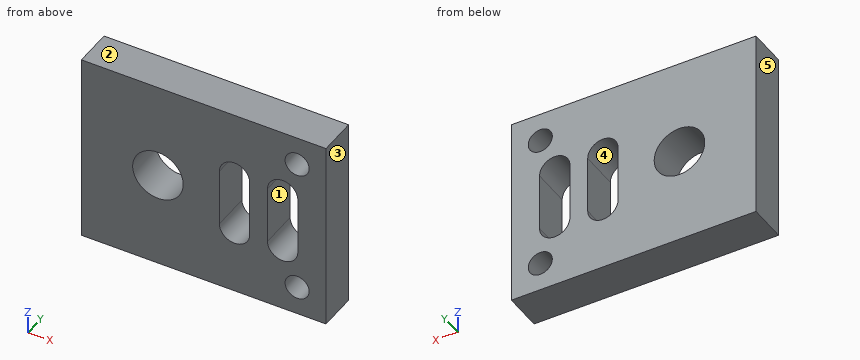
```python
from build123d import *

# Parameters (mm, degrees)
SKETCH1_W           = 25.4
SKETCH1_H           = 20
SKETCH1_R           = 1.25
SKETCH1_R_2         = 2.625
BOSS_EXTRUDE1_DEPTH = 4


with BuildPart() as part:
    # Sketch1 → Boss-Extrude1 (new body)
    with BuildSketch(Plane(origin=(0, 0, 0), x_dir=(1, 0, 0), z_dir=(0, 1, 0))):
        with Locations((12.7, 10)):
            Rectangle(SKETCH1_W, SKETCH1_H)
        with Locations((22.4, 17)):
            Circle(SKETCH1_R, mode=Mode.SUBTRACT)
        with Locations((7.95, 10)):
            Circle(SKETCH1_R_2, mode=Mode.SUBTRACT)
        with Locations((22.4, 3)):
            Circle(SKETCH1_R, mode=Mode.SUBTRACT)
        with BuildLine():
            Line((19.325, 7), (19.325, 13))
            ThreePointArc((19.325, 13), (20.9, 14.575), (22.475, 13))
            Line((22.475, 13), (22.475, 7))
            ThreePointArc((22.475, 7), (20.9, 5.425), (19.325, 7))
        make_face(mode=Mode.SUBTRACT)
        with BuildLine():
            Line((14.325, 7), (14.325, 13))
            ThreePointArc((14.325, 13), (15.9, 14.575), (17.475, 13))
            Line((17.475, 13), (17.475, 7))
            ThreePointArc((17.475, 7), (15.9, 5.425), (14.325, 7))
        make_face(mode=Mode.SUBTRACT)
    extrude(amount=-BOSS_EXTRUDE1_DEPTH)


solid = part.part
```
Design review of the part built by this model. Coordinates are the model's own, in mm. Face numbers are marked on the shaded views. A direction names the side the tool comes from. Coordinates: 2 decimals unless noted, no trailing zeros. Order: outer loops, then holes, each group sorted by start corner. A loop starts at its lowest first (then second) coordinate and runs counter-clockwise, first axis right, second up. Notation, with made-up numbers: M -2,77.5 L 29,77.5 A6 cw 29,85.5 Z; hole C 15.5,29 d5. An arc over 180 degrees is marked long. Answer as a JSON object with one key per item and string values. Group by question number.
1) Mouldability with a two-part tool opening along X and no side actions: class the marked faces 3, 4 and 5 as pulls with the +X half, pulls with the -X half, needs draft (parallel to the pull), parting line crosses it, or undercut.
2) Add section B-B, the plane y = -2.95. Write out the cut boundary in (x, z) (3 decimals), then the cut area to 3 significant figures.
3) Wall thickness on L1, parallel to X at y = -1.75, z = -10 (3 decimals); L2, parallel to Z at x = 7.95, y = -3 (3 decimals); L3, parallel to X at y = -1.3, z = -13.75: over which ranges is each line inside the solid? List them lowest first.
4) Add section A-A, the plane x = 7.95. Write out the cut boundary in (y, z) (3 decimals), then the cut area to 3 significant figures.
5) Add section C-C, the plane z = -6. Write out the cut boundary in (x, y).
6) For pin 1 (1 mm diameter, centred on x = 14, y = -3, fed in from +Z), flat-tipped, find the tip position at first contact; note if it passes through.
7) Tool access review of the marked faces 1 and 2: name each direction out of +Z, -Z, +X, -X, +Y, -Y from which nothing blocks a thin tool from reaching the whole face with its end or side.
8) Add section D-D, the plane z = -10. Write out the cut boundary in (x, y) (3 decimals), then the cut area to 3 significant figures.
Computed values:
{
 "1": {"face 3": "pulls with the +X half", "face 4": "undercut", "face 5": "pulls with the -X half"},
 "2": {"outline": "M 0,-20 L 25.4,-20 L 25.4,0 L 0,0 Z; hole C 7.95,-10 d5.25; hole M 14.325,-13 A1.575 ccw 17.475,-13 L 17.475,-7 A1.575 ccw 14.325,-7 Z; hole M 19.325,-13 A1.575 ccw 22.475,-13 L 22.475,-7 A1.575 ccw 19.325,-7 Z; hole C 22.4,-17 d2.5; hole C 22.4,-3 d2.5", "area": "423 mm^2"},
 "3": {"L1": "x = 0 to 5.325, 10.575 to 14.325, 17.475 to 19.325, 22.475 to 25.4", "L2": "z = -20 to -12.625, -7.375 to 0", "L3": "x = 0 to 14.52, 17.28 to 19.52, 22.28 to 25.4"},
 "4": {"outline": "M -4,-20 L 0,-20 L 0,-12.625 L -4,-12.625 Z; M -4,-7.375 L 0,-7.375 L 0,0 L -4,0 Z", "area": "59.0 mm^2"},
 "5": {"outline": "M 0,-4 L 14.68,-4 L 14.68,0 L 0,0 Z; M 17.12,-4 L 19.68,-4 L 19.68,0 L 17.12,0 Z; M 22.12,-4 L 25.4,-4 L 25.4,0 L 22.12,0 Z"},
 "6": {"pin 1": "stops at z = 0"},
 "7": {"face 1": "+Y, -Y", "face 2": "+Z, +X, -X, +Y, -Y"},
 "8": {"outline": "M 0,-4 L 5.325,-4 L 5.325,0 L 0,0 Z; M 10.575,-4 L 14.325,-4 L 14.325,0 L 10.575,0 Z; M 17.475,-4 L 19.325,-4 L 19.325,0 L 17.475,0 Z; M 22.475,-4 L 25.4,-4 L 25.4,0 L 22.475,0 Z", "area": "55.4 mm^2"}
}
